```python
from build123d import *

# Parameters (mm, degrees)
SKETCH1_R           = 3.1
SKETCH1_R_2         = 4.1
BOSS_EXTRUDE1_DEPTH = 3
FILLET1_R           = 3
FILLET2_R           = 1


with BuildPart() as part:
    # Sketch1 → Boss-Extrude1 (new body)
    with BuildSketch(Plane(origin=(0, 0, 0), x_dir=(1, 0, 0), z_dir=(0, 1, 0))):
        with BuildLine():
            ThreePointArc((21.667324002, 49.462380357), (-38.183766184, -38.183766184), (49.462380357, 21.667324002))
            ThreePointArc((49.462380357, 21.667324002), (46.165505457, 19.845504593), (42.585510083, 18.674162122))
            ThreePointArc((42.585510083, 18.674162122), (32.880465325, 32.880465325), (18.674162122, 42.585510083))
            ThreePointArc((18.674162122, 42.585510083), (19.845504593, 46.165505457), (21.667324002, 49.462380357))
        make_face()
        with Locations(Location((10, 0, 0), (0, 0, 270))):
            Circle(SKETCH1_R, mode=Mode.SUBTRACT)
        with Locations(Location((0, 20, 0), (0, 0, 270))):
            Circle(SKETCH1_R_2, mode=Mode.SUBTRACT)
        with Locations(Location((0, -20, 0), (0, 0, 270))):
            Circle(SKETCH1_R_2, mode=Mode.SUBTRACT)
        with Locations(Location((-10, 0, 0), (0, 0, 270))):
            Circle(SKETCH1_R, mode=Mode.SUBTRACT)
    extrude(amount=BOSS_EXTRUDE1_DEPTH)

    # Fillet1
    fillet1_edges = [part.edges().sort_by_distance(p)[0] for p in [
        (49.462380357, 1.5, -21.667324002),
        (21.667324002, 1.5, -49.462380357),
    ]]
    fillet(fillet1_edges, radius=FILLET1_R)

    # Fillet2
    fillet2_edges = [part.edges().sort_by_distance(p)[0] for p in [
        (18.674162122, 1.5, -42.585510083),
        (42.585510083, 1.5, -18.674162122),
    ]]
    fillet(fillet2_edges, radius=FILLET2_R)


solid = part.part
```
For this review, take the finished solid that the model builds, in its own axes (mm). A direction names the side the tool comes from. Round coordinates to 2 decimals unless told otherwise and drop trailing zeros. Write each loop counter-clockwise with the first axis right and the second up, starting at its lowest first coordinate (ties: lowest second). Pieces come first, ordered by that corner, then holes. Notation, with made-up numbers: (-32, -37.75) -> (-19, -37.75) arc R16 ccw to (-19, -8.75) -> close; hole circle Ø8 at (9.25, 29.5). An arc over 180 degrees is marked (long way). One line per question, with ' | ' between items. Start each with the question number.
(1) Mouldability with a two-part tool opening along Z and no side actions: class faces 1 (the face through (-1, 3, -1)), 2 (the face through (19.4, 1.48, -45.05)), 3 (the face through (-39.6, 1.48, 36.71)) as released by +Z, released by -Z, zero draft, split by the parting line, or undercut.
(2) Tool access review of faces 4 (the face through (0.18, 1.479, 15.904)), 5 (the face through (45.097, 1.479, -19.417)): name each direction out of +Z, -Z, +X, -X, +Y, -Y from which nothing blocks a thin tool from reaching the whole face with its end or side.
(3) Add section B-B, the plane z = 0. Write out the cut boundary in (x, y).
(4) Add section C-C, the plane z = 20. Write out the cut boundary in (x, y).
(5) Add section A-A, the plane x = 0. Write out the cut boundary in (y, z), plus the area to 3 significant figures.
(6) Add section D-D, the plane y = 0.55. Give the number of separate pieces and of enclosed holes in the cut face, plus the area to 3 significant figures.
(7) For line 1 along X through (y, z) = (1.85, 0); line 2 along X through (y, z) = (1.2, -20); line 3 along Z through (x, y) = (2, 1.95), list the stretches that pass through material, from the lowest coordinate up. Write a range as from..to.
(8) Insertion check: P1, Ø10, axis at x = -10, z = 0, coming from the -Y side. The pin has a flat end and moves straight along its axis. Give the tip position at first contact, or say it passes through.
Answer list:
1) face 1: zero draft | face 2: undercut | face 3: split by the parting line
2) face 4: +Y, -Y | face 5: -Z, +Y, -Y
3) outline: (-54, 0) -> (-13.1, 0) -> (-13.1, 3) -> (-54, 3) -> close; (-6.9, 0) -> (6.9, 0) -> (6.9, 3) -> (-6.9, 3) -> close; (13.1, 0) -> (54, 0) -> (54, 3) -> (13.1, 3) -> close
4) outline: (-50.16, 0) -> (-4.1, 0) -> (-4.1, 3) -> (-50.16, 3) -> close; (4.1, 0) -> (50.16, 0) -> (50.16, 3) -> (4.1, 3) -> close
5) outline: (0, -54) -> (3, -54) -> (3, -24.1) -> (0, -24.1) -> close; (0, -15.9) -> (3, -15.9) -> (3, 15.9) -> (0, 15.9) -> close; (0, 24.1) -> (3, 24.1) -> (3, 54) -> (0, 54) -> close | area: 275 mm²
6) separate pieces: 1 | enclosed holes: 4 | area: 8,710 mm²
7) line 1: -54..-13.1, -6.9..6.9, 13.1..54 | line 2: -50.16..-4.1, 4.1..41.98, 46.51..49.38 | line 3: -53.96..-23.58, -16.42..16.42, 23.58..53.96
8) P1: y = 0
